Source: CAD feature listing. Evaluate the final solid. Frame: model axes, mm. A direction names the side the tool comes from. Give positions to 0.01 mm unless a question says otherwise; leave off trailing zeros. Write each loop counter-clockwise with the first axis right and the second up, starting at its lowest first coordinate (ties: lowest second). Pieces come first, ordered by that corner, then holes. Notation, with made-up numbers: (-32, -7) -> (-21, -7) arc R37 ccw to (-21, 32) -> close; hole circle Ø2 at (-36.5, 18.25). An arc over 180 degrees is marked (long way). Use a Markdown table: item, result. Add a question column.
```python
from build123d import *

# Parameters (mm, degrees)
PLASTINA_DEPTH        = 3
OTVERSTIYA_DEPTH      = 116.156318141
OTVERSTIYA_DEPTH_BACK = 116.156318141
ESKIZ_OTVERSTIYA_R    = 1.65
ESKIZ_OTVERSTIYA_R_2  = 3.5


with BuildPart() as part:
    # Eskiz_kontur → Plastina (new body)
    with BuildSketch(Plane.XY):
        with BuildLine():
            Line((7.29115, -15.8573), (0.27924, -15.99756))
            ThreePointArc((0.27924, -15.99756), (-15.999996904, 0), (0.27924, 15.99756))
            Line((0.27924, 15.99756), (7.29115, 15.8573))
            ThreePointArc((7.29115, 15.8573), (46.200008227, 9.528004702), (85.330859965, 14.296198255))
            Line((85.330859965, 14.296198255), (100.244329965, 13.997868255))
            ThreePointArc((100.244329965, 13.997868255), (113.999902223, 0), (100.244329965, -13.997868255))
            Line((100.244329965, -13.997868255), (85.330859965, -14.296198255))
            ThreePointArc((85.330859965, -14.296198255), (46.200008227, -9.528004702), (7.29115, -15.8573))
        make_face()
        with BuildLine():
            Line((58, 3), (44, 3))
            ThreePointArc((44, 3), (41, 0), (44, -3))
            Line((44, -3), (58, -3))
            ThreePointArc((58, -3), (61, 0), (58, 3))
        make_face(mode=Mode.SUBTRACT)
    extrude(amount=PLASTINA_DEPTH)

    # Eskiz_otverstiya → Otverstiya (cut, two sides: drawn at the far end of the back side and taken through both)
    with BuildSketch(Plane.XY.offset(-OTVERSTIYA_DEPTH_BACK)):
        with Locations((-6.36396, -6.36396)):
            Circle(ESKIZ_OTVERSTIYA_R)
        with Locations((6.36396, -6.36396)):
            Circle(ESKIZ_OTVERSTIYA_R)
        Circle(ESKIZ_OTVERSTIYA_R_2)
        with Locations((35, 0)):
            Circle(ESKIZ_OTVERSTIYA_R)
        with Locations((-6.36396, 6.36396)):
            Circle(ESKIZ_OTVERSTIYA_R)
        with Locations((6.36396, 6.36396)):
            Circle(ESKIZ_OTVERSTIYA_R)
        with Locations((68, 0)):
            Circle(ESKIZ_OTVERSTIYA_R)
        with Locations((100, 0)):
            Circle(ESKIZ_OTVERSTIYA_R)
    extrude(amount=OTVERSTIYA_DEPTH + OTVERSTIYA_DEPTH_BACK, mode=Mode.SUBTRACT)


solid = part.part
```
(1) Cut plane B-B on z = 1.55. Count the separate pieces of the cut face and the enclosed holes in it, then the cut area to 3 significant figures.
(2) Access query for faces 1 (the flat face through (51, 3, 1)), 2 (the cylindrical face through (45.65, 9.54, 1.48)). Directions: +Z, -Z, +X, -X, +Y, -Y. A direction counts if a zero-diameter tool reaches every point of the face in a straight line with its end or side. Return the directions, or none.
(3) First-contact query: pin 1 Ø2 at (x, y) = (35, 0) entering from -Z; pin 2 Ø1.5 at (x, z) = (49.5, 1) entering from +Y. Flat tips, straight axial feed; report the tip coordinate or a pass-through.
(4) Material intervals for L1, parallel to X at y = 0, z = 1.7; L2, parallel to Y at x = 47, z = 0.8; L3, parallel to X at y = 2, z = 1.8, sorted ascending.
(5) Cut plane A-A on x = 35. Return the cut outline in (y, z).
(6) Cut plane C-C on x = 68. Return the cut outline in (y, z).
(7) Mould query, pull axis X, two halves, no side actions, for faces 3 (the cylindrical face through (66.784, 1.115, 1.479)), 4 (the cylindrical face through (114, 0, 1)), 5 (the flat face through (49.9, -3.3, 3)). Classes: +X half, -X half, draft (parallel to the pull), parting line (faces both ways), or undercut.
Output:
| question | item | result |
|---|---|---|
| 1 | separate pieces | 1 |
| 1 | enclosed holes | 9 |
| 1 | area | 2,920 mm^2 |
| 2 | face 1 | +Z, -Z |
| 2 | face 2 | +Z, -Z, +Y |
| 3 | pin 1 | through |
| 3 | pin 2 | y = 9.51 |
| 4 | L1 | -16 to -3.5, 3.5 to 33.35, 36.65 to 41, 61 to 66.35, 69.65 to 98.35, 101.65 to 114 |
| 4 | L2 | -9.51 to -3, 3 to 9.51 |
| 4 | L3 | -15.87 to -2.87, 2.87 to 41.76, 60.24 to 113.86 |
| 5 | outline | (-10.2, 0) -> (-1.65, 0) -> (-1.65, 3) -> (-10.2, 3) -> close; (1.65, 0) -> (10.2, 0) -> (10.2, 3) -> (1.65, 3) -> close |
| 6 | outline | (-10.8, 0) -> (-1.65, 0) -> (-1.65, 3) -> (-10.8, 3) -> close; (1.65, 0) -> (10.8, 0) -> (10.8, 3) -> (1.65, 3) -> close |
| 7 | face 3 | undercut |
| 7 | face 4 | +X half |
| 7 | face 5 | draft |
